Autodesk Inventor part; units mm, degrees
ref_plane "YZ Plane" through (0, 0, 0) normal (1, 0, 0) x (0, 1, 0)
ref_plane "XZ Plane" through (0, 0, 0) normal (0, 1, 0) x (-1, 0, 0)
ref_plane "XY Plane" through (0, 0, 0) normal (0, 0, 1) x (1, 0, 0)
ref_plane "Work Plane1" through (0, 0, 0) normal (0, 0, 1) x (1, 0, 0)
sketch "Sketch1" plane through (0, 0, 0) normal (0, 0, 1) x (1, 0, 0)
  circle A0 centre (0, 0) radius 25.6348
  circle A1 centre (0, 0) radius 12.7
  circle A2 centre (6.7, 20.6205) radius 1.5875
  circle A3 centre (17.5408, 12.7442) radius 1.5875
  circle A4 centre (21.6817, 0) radius 1.5875
  circle A5 centre (17.5408, -12.7442) radius 1.5875
  circle A6 centre (6.7, -20.6205) radius 1.5875
  circle A7 centre (-6.7, -20.6205) radius 1.5875
  circle A8 centre (-17.5408, -12.7442) radius 1.5875
  circle A9 centre (-21.6817, 0) radius 1.5875
  circle A10 centre (-17.5408, 12.7442) radius 1.5875
  circle A11 centre (-6.7, 20.6205) radius 1.5875
  point P0 (0, 0)
extrude "Extrusion1" add sketch "Sketch1" along normal blind 3.175
properties part number "basePlate" material "Polycarbonate, Clear"
For this review, take the finished solid that the model builds, in its own axes (mm). Round coordinates to 2 decimals unless told otherwise and drop trailing zeros. Loops run counter-clockwise (first coordinate to the right, second up) from the corner with the lowest first, then second, coordinate; pieces in that order, holes last.
(1) Clearance check with flat-ended pins moving along their axes: P1, Ø1.5, axis at x = 18.5, z = 2.5, coming from the +Y side; P2, Ø1.9, axis at x = 17.54, y = -12.74, coming from the -Z side; P3, Ø1.5, axis at y = -16.5, z = 0.5, coming from the +X side. State where each tip first meets the part, or that it passes through.
Returned:
P1: stops at y = 18.5
P2: passes through
P3: stops at x = 20.23
(2) Wall thickness on line 1 along Y through (x, z) = (6.7, 0.65); line 2 along X through (y, z) = (-22, 2.9); line 3 along Y through (x, z) = (0, 2.2): over which ranges is each line inside the solid? List them lowest first.
Returned:
line 1: y = -24.74 to -22.21, -19.03 to -10.79, 10.79 to 19.03, 22.21 to 24.74
line 2: x = -13.16 to -7.49, -5.91 to 5.91, 7.49 to 13.16
line 3: y = -25.63 to -12.7, 12.7 to 25.63
(3) We need section C-C (y = -6). Give the boundary of the cut face in (x, z) (3 decimals), plus the area to 3 significant figures.
Returned:
outline: (-24.923, 0) - (-11.193, 0) - (-11.193, 3.175) - (-24.923, 3.175) - close; (11.193, 0) - (24.923, 0) - (24.923, 3.175) - (11.193, 3.175) - close
area: 87.2 mm2
(4) Mouldability with a two-part tool opening along X and no side actions: class faces 1 (the flat face through (-12, -5, 0)), 2 (the cylindrical face through (-18.89, -17.33, 1.57)), 3 (the cylindrical face through (7.43, 22.03, 1.57)) as released by +X, released by -X, zero draft, split by the parting line, or undercut.
Returned:
face 1: zero draft
face 2: split by the parting line
face 3: undercut
(5) We need section B-B (x = 0). Give the boundary of the cut face in (y, z) (3 decimals).
Returned:
outline: (-25.635, 0) - (-12.7, 0) - (-12.7, 3.175) - (-25.635, 3.175) - close; (12.7, 0) - (25.635, 0) - (25.635, 3.175) - (12.7, 3.175) - close
(6) We need section D-D (x = -6.7). Give the boundary of the cut face in (y, z) (3 decimals).
Returned:
outline: (-24.744, 0) - (-22.208, 0) - (-22.208, 3.175) - (-24.744, 3.175) - close; (-19.033, 0) - (-10.789, 0) - (-10.789, 3.175) - (-19.033, 3.175) - close; (10.789, 0) - (19.033, 0) - (19.033, 3.175) - (10.789, 3.175) - close; (22.208, 0) - (24.744, 0) - (24.744, 3.175) - (22.208, 3.175) - close
(7) We need section A-A (y = 0). Give the boundary of the cut face in (x, z) (3 decimals), plus the area to 3 significant figures.
Returned:
outline: (-25.635, 0) - (-23.269, 0) - (-23.269, 3.175) - (-25.635, 3.175) - close; (-20.094, 0) - (-12.7, 0) - (-12.7, 3.175) - (-20.094, 3.175) - close; (12.7, 0) - (20.094, 0) - (20.094, 3.175) - (12.7, 3.175) - close; (23.269, 0) - (25.635, 0) - (25.635, 3.175) - (23.269, 3.175) - close
area: 62.0 mm2
